Can you work these out from the model? Positions are in its coordinate system, mm. A direction names the side the tool comes from. Give positions to 0.01 mm unless a question says otherwise; leave off trailing zeros. Order: outer loops, then holes, each group sorted by start corner. A loop starts at its lowest first (then second) coordinate and runs counter-clockwise, first axis right, second up. Notation, with made-up numbers: (-12, 48) - (17, 48) arc R26 cw to (17, 85) - close; hole circle Ø1 at (82, 80.5). An arc over 180 degrees is marked (long way). One line per question, with ' | ' between items.
```python
from build123d import *

# Parameters (mm, degrees)
SKETCH1_R             = 27.5
BOSS_EXTRUDE1_DEPTH   = 15
SKETCH2_R             = 5
CUT_EXTRUDE1_DEPTH    = 42.683330001
SKETCH3_R             = 2.534672143
CUT_EXTRUDE2_DEPTH    = 11.683899
CIRPATTERN1_START     = 3.316101093
CIRPATTERN1_OUTLINE_R = 2.534672143
CIRPATTERN1_DEPTH     = 11.683898907


# Read off the part's stored shape, not the designer's step: CirPattern1
with BuildPart() as part:
    # Sketch1 → Boss-Extrude1 (new body)
    with BuildSketch(Plane(origin=(0, 0, 0), x_dir=(1, 0, 0), z_dir=(0, 1, 0))):
        with Locations(Location((0, 0, 0), (0, 0, 270))):
            Circle(SKETCH1_R)
    extrude(amount=BOSS_EXTRUDE1_DEPTH)

    # Sketch2 → Cut-Extrude1 (cut, through all)
    with BuildSketch(Plane(origin=(0, 0, 0), x_dir=(1, 0, 0), z_dir=(0, 1, 0))):
        with Locations(Location((0, 0, 0), (0, 0, 270))):
            Circle(SKETCH2_R)
    extrude(amount=CUT_EXTRUDE1_DEPTH, mode=Mode.SUBTRACT)

    # Sketch3 → Cut-Extrude2 (cut)
    with BuildSketch(Plane(origin=(0, 15, 0), x_dir=(1, 0, 0), z_dir=(0, 1, 0))):
        with Locations(Location((-9.347834619, 0, 0), (0, 0, 270))):
            Circle(SKETCH3_R)
    extrude(amount=-CUT_EXTRUDE2_DEPTH, mode=Mode.SUBTRACT)

    # CirPattern1 outline → CirPattern1 (cut)
    with BuildSketch(Plane(origin=(0, 0, 0), x_dir=(1, 0, 0), z_dir=(0, 1, 0)).offset(CIRPATTERN1_START)):
        with Locations((0, 9.347834619)):
            Circle(CIRPATTERN1_OUTLINE_R)
        with Locations((9.347834619, 0)):
            Circle(CIRPATTERN1_OUTLINE_R)
        with Locations((0, -9.347834619)):
            Circle(CIRPATTERN1_OUTLINE_R)
    extrude(amount=CIRPATTERN1_DEPTH, mode=Mode.SUBTRACT)


solid = part.part
```
(1) If we mould it in two halves opening along X, with no side actions, what happens to faces 1 (the face through (-24.397, 7.395, 12.69)), 2 (the face through (-6, 15, 0)), 3 (the face through (11.765, 9.076, -0.761))? For each: released by +X, released by -X, zero draft, split by the parting line, or undercut.
Answer below:
face 1: split by the parting line | face 2: zero draft | face 3: undercut
(2) Imagine slicing it at D-D (x = 7.5). List the corners of the cut face in (y, z) for me, and give its area (3 significant figures).
Answer below:
outline: (0, -26.46) - (15, -26.46) - (15, -1.73) - (3.32, -1.73) - (3.32, 1.73) - (15, 1.73) - (15, 26.46) - (0, 26.46) - close | area: 753 mm^2
(3) Imagine slicing it at B-B (x = 0). List the corners of the cut face in (y, z) for me, and give its area (3 significant figures).
Answer below:
outline: (0, -27.5) - (15, -27.5) - (15, -11.88) - (3.32, -11.88) - (3.32, -6.81) - (15, -6.81) - (15, -5) - (0, -5) - close; (0, 5) - (15, 5) - (15, 6.81) - (3.32, 6.81) - (3.32, 11.88) - (15, 11.88) - (15, 27.5) - (0, 27.5) - close | area: 557 mm^2
(4) Imagine slicing it at C-C (y = 14). List the corners of the cut face in (x, z) for me, and give its area (3 significant figures).
Answer below:
outline: circle Ø55 at (0, 0); hole circle Ø5.07 at (-9.35, 0); hole circle Ø10 at (0, 0); hole circle Ø5.07 at (0, -9.35); hole circle Ø5.07 at (0, 9.35); hole circle Ø5.07 at (9.35, 0) | area: 2,220 mm^2
(5) If I drill on line 1 (X direction, y = 6, z = 0); line 2 (Z direction, x = 1, y = 5.75); line 3 (Y direction, x = 0.5, z = 8), over which ranges is the centre line in solid material (lowest first)?
Answer below:
line 1: -27.5 to -11.88, -6.81 to -5, 5 to 6.81, 11.88 to 27.5 | line 2: -27.48 to -11.68, -7.02 to -4.9, 4.9 to 7.02, 11.68 to 27.48 | line 3: 0 to 3.32
(6) Imagine slicing it at A-A (z = 0). List the corners of the cut face in (x, y) for me.
Answer below:
outline: (-27.5, 0) - (-5, 0) - (-5, 15) - (-6.81, 15) - (-6.81, 3.32) - (-11.88, 3.32) - (-11.88, 15) - (-27.5, 15) - close; (5, 0) - (27.5, 0) - (27.5, 15) - (11.88, 15) - (11.88, 3.32) - (6.81, 3.32) - (6.81, 15) - (5, 15) - close
(7) Will these pins go through, and if not, where does the flat tip stop? pin 1 (1 mm diameter, centred on x = 11.5, y = 3.5, fed in from -Z); pin 2 (1 mm diameter, centred on x = -6, y = 11, fed in from +Z); pin 3 (1.5 mm diameter, centred on x = -1, z = 10.5, fed in from +Y).
Answer below:
pin 1: z = -25.2 | pin 2: z = 26.94 | pin 3: y = 3.32
(8) On a 3-axis mill with a long thin cutter (end or side, diameter ignored), from which of +Z, -Z, +X, -X, +Y, -Y can I reach the whole of each face in a straight line? I mean faces 4 (the face through (9, 3.316, 0)), 5 (the face through (-4.88, 7.4, -1.08)). Say none if no direction works.
Answer below:
face 4: +Y | face 5: +Y, -Y
